For this review, take the finished solid that the model builds, in its own axes (mm). A direction names the side the tool comes from. Round coordinates to 2 decimals unless told otherwise and drop trailing zeros. Loops run counter-clockwise (first coordinate to the right, second up) from the corner with the lowest first, then second, coordinate; pieces in that order, holes last.
1. Tool access review of faces 1 (the flat face through (-3, -7.938, 30)), 2 (the flat face through (22.225, 17, 18)), 3 (the flat face through (46, -25.4, 42)): name each direction out of +Z, -Z, +X, -X, +Y, -Y from which nothing blocks a thin tool from reaching the whole face with its end or side.
2. Consider section C-C on x = 95.5. State the section outline as (y, z) points (3 decimals), then the cut area to 3 significant figures.
3. To check wall thickness, follow line 1 along Z through (x, y) = (1.5, 36.5) (3 decimals); line 2 along Y through (x, z) = (3, 30); line 3 along X through (y, z) = (13.5, 20.5) (3 decimals). State the ranges of each line that lie inside material, in increasing order.
4. Consider section B-B on x = 72.5. State the section outline as (y, z) points (3 decimals), then the cut area to 3 significant figures.
5. Draft analysis for pull direction Z (two halves, no side actions). For faces 4 (the cylindrical face through (31.92, 16.55, 51.15)), 5 (the flat face through (-3, 7.938, 30)), 6 (the flat face through (86, 0, 38.1)), state which applies: released by +Z, released by -Z, zero draft, split by the parting line, or undercut.
6. Clearance check with flat-ended pins moving along their axes: pin 1 Ø2 at (x, z) = (76, 54.5) entering from -Y; pin 2 Ø4 at (x, y) = (-11.5, -1.5) entering from +Z; pin 3 Ø5 at (y, z) = (19.5, 14) entering from -X (3 decimals). State where each tip first meets the part, or that it passes through.
7. Consider section A-A on y = 32. State the section outline as (x, z) points (3 decimals), then the cut area to 3 significant figures.
from build123d import *

# Parameters (mm, degrees)
F1_DEPTH = 63.5
F2_DEPTH = 25.4
F0_W     = 25.4
F0_H     = 19.05
F3_DEPTH = 25.4
F4_DEPTH = 7.9375
F6_R     = 6.35


with BuildPart() as f1:
    # F0 (on Front) → F1 (new body, symmetric)
    with BuildSketch(Plane.XZ):
        Polygon((-41.275, -9.525), (41.275, -9.525), (41.275, 9.525), (22.225, 9.525), (-41.275, 9.525), align=None)
    extrude(amount=F1_DEPTH, both=True)

    # F0 (on Front) → F2 (join, symmetric)
    with BuildSketch(Plane.XZ):
        with BuildLine():
            Line((22.225, 9.525), (41.275, 9.525))
            Line((41.275, 9.525), (41.275, 27.0002))
            ThreePointArc((41.275, 27.0002), (45.9246798487, 38.2255201513), (57.15, 42.8752))
            Line((57.15, 42.8752), (60.325, 42.8752))
            Line((60.325, 42.8752), (60.325, 61.9252))
            Line((60.325, 61.9252), (57.15, 61.9252))
            add(Edge.make_bspline(
                [(54.8989749886, 61.8525817177), (55.6472993307, 61.8814662978), (56.3976709314, 61.9056929595), (57.15, 61.9252)],
                knots=[109.9134052924, 109.9134052924, 109.9134052924, 109.9134052924, 111.5045361635, 111.5045361635, 111.5045361635, 111.5045361635], degree=3))
            ThreePointArc((54.8989749886, 61.8525817177), (31.6708646779, 50.8867922274), (22.225, 27.0002))
            Line((22.225, 27.0002), (22.225, 9.525))
        make_face()
    extrude(amount=F2_DEPTH, both=True)

    # F0 (on Front) → F3 (join, symmetric)
    with BuildSketch(Plane.XZ):
        with Locations((73.025, 52.4002)):
            Rectangle(F0_W, F0_H)
    extrude(amount=F3_DEPTH, both=True)

    # F0 (on Front) → F4 (join, symmetric)
    with BuildSketch(Plane.XZ):
        with BuildLine():
            add(Edge.make_bspline(
                [(-41.275, 9.525), (-38.7184419076, 35.6349297133), (3.2056302131, 59.8572696967), (54.8989749886, 61.8525817177)],
                knots=[0, 0, 0, 0, 109.9134052924, 109.9134052924, 109.9134052924, 109.9134052924], degree=3))
            Line((-41.275, 9.525), (22.225, 9.525))
            Line((22.225, 9.525), (22.225, 27.0002))
            ThreePointArc((22.225, 27.0002), (31.6708646779, 50.8867922274), (54.8989749886, 61.8525817177))
        make_face()
    extrude(amount=F4_DEPTH, both=True)

    # F0 (on Front) → F5 (revolve)
    with BuildSketch(Plane.XZ):
        Polygon((85.725, 61.9252), (85.725, 42.8752), (85.725, 38.1), (111.125, 38.1), (111.125, 66.675), (85.725, 66.675), align=None)
    revolve(axis=Axis((85.725, 0, 52.3875), (0, 0, 1)))

    # F6
    f6_edges = [f1.edges().sort_by_distance(p)[0] for p in [
        (-41.275, -63.5, 0),
        (41.275, -63.5, 0),
        (41.275, 63.5, 0),
        (-41.275, 63.5, 0),
    ]]
    fillet(f6_edges, radius=F6_R)


solid = f1.part
Resolved:
1. face 1: +Z, -X, -Y
1. face 2: +Z, -X, +Y
1. face 3: +Z, +X, -X, -Y
2. outline: (-23.444, 38.1) - (23.444, 38.1) - (23.444, 66.675) - (-23.444, 66.675) - close
2. area: 1,340 mm2
3. line 1: z = -9.525 to 9.525
3. line 2: y = -7.94 to 7.94
3. line 3: x = 22.225 to 41.275
4. outline: (-25.4, 42.875) - (-21.685, 42.875) - (-21.685, 38.1) - (21.685, 38.1) - (21.685, 42.875) - (25.4, 42.875) - (25.4, 61.925) - (21.685, 61.925) - (21.685, 66.675) - (-21.685, 66.675) - (-21.685, 61.925) - (-25.4, 61.925) - close
4. area: 1,380 mm2
5. face 4: released by +Z
5. face 5: zero draft
5. face 6: released by -Z
6. pin 1: stops at y = -25.4
6. pin 2: stops at z = 45.87
6. pin 3: stops at x = 22.225
7. outline: (-41.275, -9.525) - (41.275, -9.525) - (41.275, 9.525) - (-41.275, 9.525) - close
7. area: 1,570 mm2
